```python
from build123d import *

# Parameters (mm, degrees)
SKETCH_1_W            = 166
SKETCH_1_H            = 78
EXTRUDE_293_DEPTH     = 8
SKETCH_2_W            = 163
SKETCH_2_H            = 72
CUT_EXTRUDE_531_DEPTH = 6
SKETCH_7_W            = 163
SKETCH_7_H            = 2.2
CUT_EXTRUDE_3_DEPTH   = 1.2
SKETCH_8_W            = 75.4
SKETCH_8_H            = 2.189311695
CUT_EXTRUDE_4_DEPTH   = 2.2
SKETCH_9_W            = 163
SKETCH_9_H            = 2.2
CUT_EXTRUDE_5_DEPTH   = 1.2
SKETCH_10_W           = 2.869065247
SKETCH_10_H           = 72
EXTRUDE_1_DEPTH       = 2


with BuildPart() as part:
    # Эскиз1 → Extrude 293 (new body)
    with BuildSketch(Plane(origin=(0, 0, 0), x_dir=(1, 0, 0), z_dir=(0, 1, 0))):
        with Locations((83, 39)):
            Rectangle(SKETCH_1_W, SKETCH_1_H)
    extrude(amount=EXTRUDE_293_DEPTH)

    # Эскиз2 → Cut-Extrude 531 (cut)
    with BuildSketch(Plane(origin=(0, 8, 0), x_dir=(1, 0, 0), z_dir=(0, 1, 0))):
        with Locations((84.5, 39)):
            Rectangle(SKETCH_2_W, SKETCH_2_H)
    extrude(amount=-CUT_EXTRUDE_531_DEPTH, mode=Mode.SUBTRACT)

    # Эскиз7 → Вырез-Вытянуть3 (cut)
    with BuildSketch(Plane.XY.offset(-75)):
        with Locations((84.5, 5.1)):
            Rectangle(SKETCH_7_W, SKETCH_7_H)
    extrude(amount=-CUT_EXTRUDE_3_DEPTH, mode=Mode.SUBTRACT)

    # Эскиз8 → Вырез-Вытянуть4 (cut)
    with BuildSketch(Plane(origin=(3, 0, 0), x_dir=(0, 0, -1), z_dir=(1, 0, 0))):
        with Locations((38.5, 5.105344153)):
            Rectangle(SKETCH_8_W, SKETCH_8_H)
    extrude(amount=-CUT_EXTRUDE_4_DEPTH, mode=Mode.SUBTRACT)

    # Эскиз9 → Вырез-Вытянуть5 (cut)
    with BuildSketch(Plane(origin=(0, 0, -3), x_dir=(-1, 0, 0), z_dir=(0, 0, -1))):
        with Locations((-84.5, 5.1)):
            Rectangle(SKETCH_9_W, SKETCH_9_H)
    extrude(amount=-CUT_EXTRUDE_5_DEPTH, mode=Mode.SUBTRACT)

    # Эскиз10 → Бобышка-Вытянуть1 (add)
    with BuildSketch(Plane(origin=(0, 2, 0), x_dir=(1, 0, 0), z_dir=(0, 1, 0))):
        with Locations((164.565467377, 39)):
            Rectangle(SKETCH_10_W, SKETCH_10_H)
    extrude(amount=EXTRUDE_1_DEPTH)


solid = part.part
```
The model under review builds one solid part; all positions refer to its coordinate system, in mm. Give positions to 0.01 mm unless a question says otherwise; leave off trailing zeros. Write each loop counter-clockwise with the first axis right and the second up, starting at its lowest first coordinate (ties: lowest second). Pieces come first, ordered by that corner, then holes. Notation, with made-up numbers: M 18,-3.75 L 45,-3.75 A24 ccw 45,7.25 Z; hole C 37.5,81 d7. An arc over 180 degrees is marked long. Answer in a Markdown table with one row per item.
Item 1: Add section A-A on x = 100. Give the boundary of the cut face in (y, z), plus the area to 3 significant figures.
Check sheet entries:
| item | result |
|---|---|
| outline | M 0,-78 L 8,-78 L 8,-75 L 6.2,-75 L 6.2,-76.2 L 4,-76.2 L 4,-75 L 2,-75 L 2,-3 L 4,-3 L 4,-1.8 L 6.2,-1.8 L 6.2,-3 L 8,-3 L 8,0 L 0,0 Z |
| area | 187 mm2 |
Item 2: Add section B-B on z = -20.5. Give the boundary of the cut face in (x, y), plus the area to 3 significant figures.
Check sheet entries:
| item | result |
|---|---|
| outline | M 0,0 L 166,0 L 166,4 L 163.13,4 L 163.13,2 L 3,2 L 3,4.01 L 0.8,4.01 L 0.8,6.2 L 3,6.2 L 3,8 L 0,8 Z |
| area | 351 mm2 |
Item 3: For P1, Ø3, axis at x = 101, z = -62.5, coming from the +Y side; P2, Ø1.1, axis at y = 5, z = -22.5, coming from the +X side, all flat-tipped, find the tip position at first contact; note any pin that passes through.
Check sheet entries:
| item | result |
|---|---|
| P1 | y = 2 |
| P2 | x = 0.8 |
Item 4: For line 1 along X through (y, z) = (2.5, -8.5); line 2 along Z through (x, y) = (154.5, 4.75); line 3 along Z through (x, y) = (19.5, 3.5), list the stretches that pass through material, from the lowest coordinate up.
Check sheet entries:
| item | result |
|---|---|
| line 1 | 0 to 3, 163.13 to 166 |
| line 2 | -78 to -76.2, -1.8 to 0 |
| line 3 | -78 to -75, -3 to 0 |
Item 5: Draft analysis for pull direction X (two halves, no side actions). For faces 1 (the face through (82, 2, -40)), 2 (the face through (166, 2, -38)), 3 (the face through (82, 4, 0)), state which applies: +X half, -X half, draft (parallel to the pull), parting line (faces both ways), or undercut.
Check sheet entries:
| item | result |
|---|---|
| face 1 | undercut |
| face 2 | +X half |
| face 3 | draft |
